```python
from build123d import *

# Parameters (mm, degrees)
F1_DEPTH = 5.08


with BuildPart() as f1:
    # F0 (on Front) → F1 (new body)
    with BuildSketch(Plane.XZ):
        with BuildLine():
            Line((-2.331354, 19.470736), (-2.331354, 0))
            ThreePointArc((-2.331354, 0), (-9.180507, -4.784652), (-10.948811, -12.950245))
            ThreePointArc((-10.948811, -12.950245), (-9.562296, -14.777595), (-7.400639, -15.544976))
            ThreePointArc((-7.400639, -15.544976), (-4.957759, -14.557545), (-5.236087, -11.937389))
            ThreePointArc((-5.236087, -11.937389), (-7.423099, -9.830791), (-6.679121, -6.886768))
            ThreePointArc((-6.679121, -6.886768), (-4.067414, -3.763698), (0, -3.588403))
            ThreePointArc((0, -3.588403), (4.067414, -3.763698), (6.679121, -6.886768))
            ThreePointArc((6.679121, -6.886768), (7.423099, -9.830791), (5.236087, -11.937389))
            ThreePointArc((5.236087, -11.937389), (4.957759, -14.557545), (7.400639, -15.544976))
            ThreePointArc((7.400639, -15.544976), (9.562296, -14.777595), (10.948811, -12.950245))
            ThreePointArc((10.948811, -12.950245), (9.180507, -4.784652), (2.331354, 0))
            Line((2.331354, 0), (2.331354, 19.470736))
            Line((2.331354, 19.470736), (0, 19.470736))
            Line((0, 19.470736), (-2.331354, 19.470736))
        make_face()
    extrude(amount=F1_DEPTH)


solid = f1.part
```
Input: part model. Units: mm. Frame: model coordinates. A direction names the side the tool comes from. Round coordinates to 2 decimals unless told otherwise and drop trailing zeros. Loops run counter-clockwise (first coordinate to the right, second up) from the corner with the lowest first, then second, coordinate; pieces in that order, holes last. Notation, with made-up numbers: (58, -39.75) -> (106, -39.75) arc R19 cw to (106, -19.75) -> close; hole circle Ø3 at (81, 21.25). An arc over 180 degrees is marked (long way). Use one line per item in the form item = value. Start each with the question number.
Item 1: Section query B-B on z = 13. Return the cut outline in (x, y).
Item 2: Section query C-C on y = -4.65. Return the cut outline in (x, z), then the cut area to 3 significant figures.
Item 3: Material intervals for L1, parallel to X at y = -0.85, z = 16; L2, parallel to X at y = -4.8, z = -4; L3, parallel to X at y = -3.55, z = -10, sorted ascending. Write a range as from..to.
Item 4: Section query D-D on z = -10. Return the cut outline in (x, y), then the cut area to 3 significant figures.
Item 5: Set-up query: faces 1 (the face through (-2.331, -3, 10)), 2 (the face through (-4.12, -2.5, -3.79)), 3 (the face through (2.331, -3, 10)). Return all of +Z, -Z, +X, -X, +Y, -Y with unobstructed straight access to the full face (end or side cutting, diameter ignored); none if empty.
Item 6: Section query A-A on z = -5.5. Return the cut outline in (x, y), then the cut area to 3 significant figures.
Item 7: Mould query, pull axis Z, two halves, no side actions, for faces 4 (the face through (1, -5.08, -2)), 5 (the face through (-9.589, -2.504, -14.758)), 6 (the face through (4.938, -2.504, -14.523)). Classes: pulls with the +Z half, pulls with the -Z half, needs draft (parallel to the pull), parting line crosses it, or undercut.
Ans:
q1.outline = (-2.33, -5.08) -> (2.33, -5.08) -> (2.33, 0) -> (-2.33, 0) -> close
q2.outline = (-10.95, -12.95) arc R4.01 ccw to (-7.4, -15.54) arc R2.19 ccw to (-5.24, -11.94) arc R3.02 cw to (-6.68, -6.89) arc R5.04 cw to (0, -3.59) arc R5.04 cw to (6.68, -6.89) arc R3.02 cw to (5.24, -11.94) arc R2.19 ccw to (7.4, -15.54) arc R4.01 ccw to (10.95, -12.95) arc R11.44 ccw to (2.33, 0) -> (2.33, 19.47) -> (-2.33, 19.47) -> (-2.33, 0) arc R11.44 ccw to start
q2.area = 233 mm^2
q3.L1 = -2.33..2.33
q3.L2 = -8.61..-4.49, 4.49..8.61
q3.L3 = -11.04..-7.37, 7.37..11.04
q4.outline = (-11.04, -5.08) -> (-7.37, -5.08) -> (-7.37, 0) -> (-11.04, 0) -> close; (7.37, -5.08) -> (11.04, -5.08) -> (11.04, 0) -> (7.37, 0) -> close
q4.area = 37.3 mm^2
q5.face_1 = +Z, -X, +Y, -Y
q5.face_2 = +Y, -Y
q5.face_3 = +Z, +X, +Y, -Y
q6.outline = (-9.62, -5.08) -> (-6.04, -5.08) -> (-6.04, 0) -> (-9.62, 0) -> close; (6.04, -5.08) -> (9.62, -5.08) -> (9.62, 0) -> (6.04, 0) -> close
q6.area = 36.4 mm^2
q7.face_4 = needs draft
q7.face_5 = pulls with the -Z half
q7.face_6 = undercut
